Part model, mm, in its own coordinate system. Face numbers are marked on the shaded views. A direction names the side the tool comes from. Give positions to 0.01 mm unless a question says otherwise; leave off trailing zeros. Write each loop counter-clockwise with the first axis right and the second up, starting at its lowest first coordinate (ties: lowest second). Pieces come first, ordered by that corner, then holes. Notation, with made-up numbers: M 85.25,52 L 134.25,52 A5 cw 134.25,61 Z; hole C 78,61.5 d8. An arc over 180 degrees is marked long. Answer as CSV lines item,"result". Start each with the question number.
Item 1: Band-saw the part on B-B, the plane z = -3. List the corners of the cut face in (x, y), then the cut area to 3 significant figures.
Item 2: Two-plate mould, pull along Y, no slides. Class the marked faces 1, 2 and 3: +Y half, -Y half, draft (parallel to the pull), parting line (faces both ways), or undercut.
Item 3: Band-saw the part on A-A, the plane y = 0. List the corners of the cut face in (x, z).
Item 4: 3-axis set-ups, long thin cutter, end or side, ignore diameter. For the marked faces 4, 5 and 6: which of +Z, -Z, +X, -X, +Y, -Y reach the whole face in a straight line?
Item 5: Pin check, flat tips, straight feed: pin 1 (1.5 mm diameter, centred on x = 7.5, z = 15.5, fed in from +Y); pin 2 (14 mm diameter, centred on x = 0, y = 0, fed in from -Z); pin 3 (6 mm diameter, centred on x = 3, y = -0.5, fed in from -Z). Stop position of each tip, or through.
Item 6: Wall check: L1, parallel to X at y = 9.3, z = 15; L2, parallel to X at y = 0, z = -8.5; L3, parallel to Y at x = -0.25, z = 8. Give the ranges that are in metal, low to high. Write a range as from..to.
Item 7: Band-saw the part on D-D, the plane z = -15. List the corners of the cut face in (x, y).
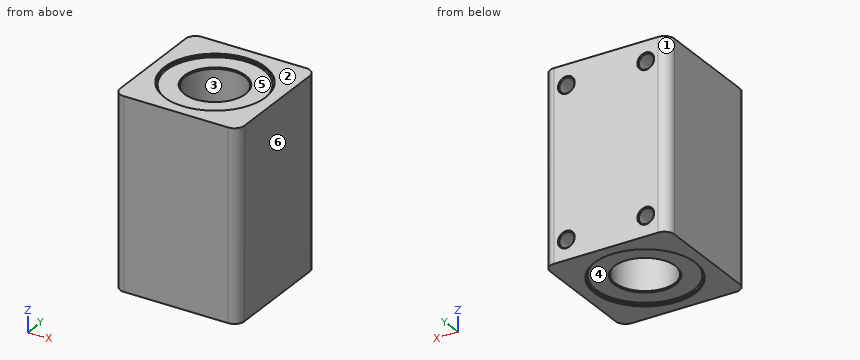
from build123d import *

# Parameters (mm, degrees)
SKETCH1_W          = 25
SKETCH1_H          = 25
SKETCH1_R          = 6
BASE_EXTRUDE_DEPTH = 19
SKETCH2_R          = 10
FRONTDETAIL_DEPTH  = 0.5
FILLET1_R          = 2
SKETCH3_R          = 1.5
MOUNTS_DEPTH       = 4.5
CHAMFER1_SIZE      = 0.2


with BuildPart() as part:
    # Sketch1 → Base-Extrude (new, symmetric)
    with BuildSketch(Plane.XY):
        Rectangle(SKETCH1_W, SKETCH1_H)
        Circle(SKETCH1_R, mode=Mode.SUBTRACT)
    extrude(amount=BASE_EXTRUDE_DEPTH, both=True)

    # Sketch2 → FrontDetail (cut)
    with BuildSketch(Plane.XY.offset(19)):
        Circle(SKETCH2_R)
    frontdetail = extrude(amount=-FRONTDETAIL_DEPTH, mode=Mode.SUBTRACT)

    # Mirror1: FrontDetail across plane
    add(frontdetail.mirror(Plane.XY), mode=Mode.SUBTRACT)

    # Fillet1
    fillet1_edges = [part.edges().sort_by_distance(p)[0] for p in [
        (-12.5, 12.5, 0),
        (12.5, 12.5, 0),
        (12.5, -12.5, 0),
        (-12.5, -12.5, 0),
    ]]
    fillet(fillet1_edges, radius=FILLET1_R)

    # Sketch3 → Mounts (cut)
    with BuildSketch(Plane(origin=(0, 12.5, 0), x_dir=(-1, 0, 0), z_dir=(0, 1, 0))):
        with Locations(Location((-8, 15, 0), (0, 0, 90))):
            Circle(SKETCH3_R)
        with Locations(Location((8, 15, 0), (0, 0, 90))):
            Circle(SKETCH3_R)
        with Locations(Location((-8, -15, 0), (0, 0, 90))):
            Circle(SKETCH3_R)
        with Locations(Location((8, -15, 0), (0, 0, 90))):
            Circle(SKETCH3_R)
    extrude(amount=-MOUNTS_DEPTH, mode=Mode.SUBTRACT)

    # Chamfer1
    chamfer1_edges = [part.edges().sort_by_distance(p)[0] for p in [
        (-10, 0, 18.5),
        (-6, 0, 18.5),
        (-10, 0, 19),
        (-10, 0, -19),
        (-6, 0, -18.5),
        (-10, 0, -18.5),
        (8, 12.5, 13.5),
        (-8, 12.5, 13.5),
        (8, 12.5, -16.5),
        (-8, 12.5, -16.5),
    ]]
    chamfer(chamfer1_edges, length=CHAMFER1_SIZE)


solid = part.part
Output:
1,outline,"M -12.5,-10.5 A2 ccw -10.5,-12.5 L 10.5,-12.5 A2 ccw 12.5,-10.5 L 12.5,10.5 A2 ccw 10.5,12.5 L -10.5,12.5 A2 ccw -12.5,10.5 Z; hole C 0,0 d12"
1,area,"508 mm²"
2,face 1,"+Y half"
2,face 2,"draft"
2,face 3,"undercut"
3,outline,"M -12.5,-19 L -10.2,-19 L -10,-18.8 L -10,-18.7 L -9.8,-18.5 L -6.2,-18.5 L -6,-18.3 L -6,18.3 L -6.2,18.5 L -9.8,18.5 L -10,18.7 L -10,18.8 L -10.2,19 L -12.5,19 Z; M 6,-18.3 L 6.2,-18.5 L 9.8,-18.5 L 10,-18.7 L 10,-18.8 L 10.2,-19 L 12.5,-19 L 12.5,19 L 10.2,19 L 10,18.8 L 10,18.7 L 9.8,18.5 L 6.2,18.5 L 6,18.3 Z"
4,face 4,"-Z"
4,face 5,"+Z"
4,face 6,"+Z, -Z, +X, +Y, -Y"
5,pin 1,"y = 8"
5,pin 2,"z = -18.5"
5,pin 3,"z = -18.34"
6,L1,"-12.5..-9.5, -6.5..6.5, 9.5..12.5"
6,L2,"-12.5..-6, 6..12.5"
6,L3,"-12.5..-5.99, 5.99..12.5"
7,outline,"M -12.5,-10.5 A2 ccw -10.5,-12.5 L 10.5,-12.5 A2 ccw 12.5,-10.5 L 12.5,10.5 A2 ccw 10.5,12.5 L 9.7,12.5 L 9.5,12.3 L 9.5,8 L 6.5,8 L 6.5,12.3 L 6.3,12.5 L -6.3,12.5 L -6.5,12.3 L -6.5,8 L -9.5,8 L -9.5,12.3 L -9.7,12.5 L -10.5,12.5 A2 ccw -12.5,10.5 Z; hole C 0,0 d12"
